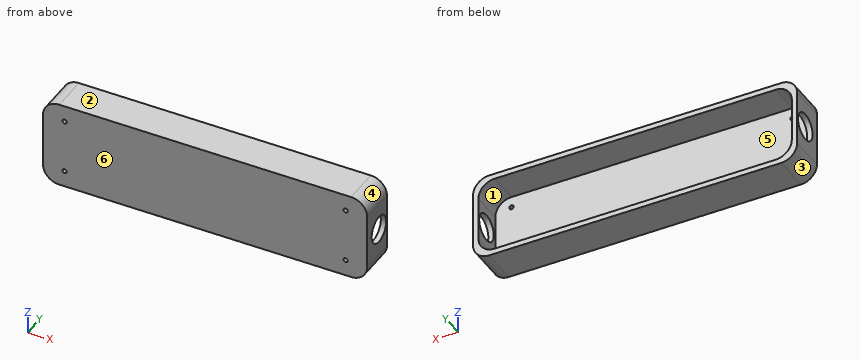
from build123d import *

# Parameters (mm, degrees)
SKETCH1_W               = 300
SKETCH1_H               = 80.5
SKETCH1_W_2             = 290
SKETCH1_H_2             = 70.5
BOSS_EXTRUDE1_DEPTH     = 34
SKETCH1_3_W             = 290
SKETCH1_3_H             = 70.5
BOSS_EXTRUDE2_DEPTH     = 5
FILLET1_R               = 15
FILLET2_R               = 15
FILLET3_R               = 15
FILLET4_R               = 15
FILLET5_R               = 15
FILLET6_R               = 15
FILLET7_R               = 15
FILLET8_R               = 15
SKETCH2_R               = 2
CUT_EXTRUDE1_DEPTH      = 159.984472512
MIRROR2_COPY_1_SKETCH_R = 2
MIRROR2_COPY_1_DEPTH    = 159.984472512
SKETCH3_R               = 12.5
CUT_EXTRUDE2_DEPTH      = 305.591632354


with BuildPart() as part:
    # Sketch1 → Boss-Extrude1 (new body)
    with BuildSketch(Plane(origin=(0, 0, 0), x_dir=(1, 0, 0), z_dir=(0, 1, 0))):
        Rectangle(SKETCH1_W, SKETCH1_H)
        Rectangle(SKETCH1_W_2, SKETCH1_H_2, mode=Mode.SUBTRACT)
    extrude(amount=BOSS_EXTRUDE1_DEPTH)

    # Sketch1_3 → Boss-Extrude2 (add)
    with BuildSketch(Plane(origin=(0, 0, 0), x_dir=(1, 0, 0), z_dir=(0, 1, 0))):
        Rectangle(SKETCH1_3_W, SKETCH1_3_H)
    extrude(amount=BOSS_EXTRUDE2_DEPTH)

    # Fillet1
    fillet1_edges = [part.edges().sort_by_distance(p)[0] for p in [
        (-150, 17, 40.25),
    ]]
    fillet(fillet1_edges, radius=FILLET1_R)

    # Fillet2
    fillet2_edges = [part.edges().sort_by_distance(p)[0] for p in [
        (-150, 17, -40.25),
    ]]
    fillet(fillet2_edges, radius=FILLET2_R)

    # Fillet3
    fillet3_edges = [part.edges().sort_by_distance(p)[0] for p in [
        (150, 17, -40.25),
    ]]
    fillet(fillet3_edges, radius=FILLET3_R)

    # Fillet4
    fillet4_edges = [part.edges().sort_by_distance(p)[0] for p in [
        (150, 17, 40.25),
    ]]
    fillet(fillet4_edges, radius=FILLET4_R)

    # Fillet5
    fillet5_edges = [part.edges().sort_by_distance(p)[0] for p in [
        (-145, 19.5, -35.25),
    ]]
    fillet(fillet5_edges, radius=FILLET5_R)

    # Fillet6
    fillet6_edges = [part.edges().sort_by_distance(p)[0] for p in [
        (-145, 19.5, 35.25),
    ]]
    fillet(fillet6_edges, radius=FILLET6_R)

    # Fillet7
    fillet7_edges = [part.edges().sort_by_distance(p)[0] for p in [
        (145, 19.5, -35.25),
    ]]
    fillet(fillet7_edges, radius=FILLET7_R)

    # Fillet8
    fillet8_edges = [part.edges().sort_by_distance(p)[0] for p in [
        (145, 19.5, 35.25),
    ]]
    fillet(fillet8_edges, radius=FILLET8_R)

    # Sketch2 → Cut-Extrude1 (cut, through all)
    with BuildSketch(Plane(origin=(0, 0, 0), x_dir=(-1, 0, 0), z_dir=(0, -1, 0))):
        with Locations(Location((-130, -25, 0), (0, 0, 90))):
            Circle(SKETCH2_R)
    cut_extrude1 = extrude(amount=-CUT_EXTRUDE1_DEPTH, mode=Mode.SUBTRACT)

    # Mirror1: Cut-Extrude1 across plane
    add(cut_extrude1.mirror(Plane.XY), mode=Mode.SUBTRACT)

    # Mirror2: Cut-Extrude1 across plane
    add(cut_extrude1.mirror(Plane(origin=(0, 0, 0), x_dir=(0, 0, 1), z_dir=(1, 0, 0))), mode=Mode.SUBTRACT)

    # Mirror2 copy 1 sketch → Mirror2 copy 1 (cut, through all)
    with BuildSketch(Plane.XZ):
        with Locations(Location((-130, -25, 0), (0, 0, 90))):
            Circle(MIRROR2_COPY_1_SKETCH_R)
    extrude(amount=-MIRROR2_COPY_1_DEPTH, mode=Mode.SUBTRACT)

    # Sketch3 → Cut-Extrude2 (cut, through all)
    with BuildSketch(Plane(origin=(150, 0, 0), x_dir=(0, 0, -1), z_dir=(1, 0, 0))):
        with Locations((0, 20.125)):
            Circle(SKETCH3_R)
    extrude(amount=-CUT_EXTRUDE2_DEPTH, mode=Mode.SUBTRACT)


solid = part.part
Verification items for the finished model (mm, model axes). Face numbers are marked on the shaded views. A direction names the side the tool comes from. Round coordinates to 2 decimals unless told otherwise and drop trailing zeros. Loops run counter-clockwise (first coordinate to the right, second up) from the corner with the lowest first, then second, coordinate; pieces in that order, holes last. Notation, with made-up numbers: (84.25, 85.5) - (102.25, 85.5) arc R26 cw to (102.25, 116.5) - close; hole circle Ø3 at (14, -35.75). An arc over 180 degrees is marked (long way). Answer in a Markdown table with one row per item. Add a question column.
Q1. Tool access check on the marked faces 5 and 6. Record the directions out of +Z, -Z, +X, -X, +Y, -Y that give a thin tool (end or side, any length) a straight path to the whole face; none if there is none.
Q2. Gauge pin test, flat ends, axial feed: pin 1 (1.5 mm diameter, centred on y = 4, z = -31.5, fed in from +X); pin 2 (21 mm diameter, centred on x = -13.5, z = -11, fed in from +Y); pin 3 (3.5 mm diameter, centred on x = -130, z = 25, fed in from +Y). Record the tip position at first contact, or that the pin passes through.
Q3. Section check C-C on y = 12. Enter the section's corners in (x, z), plus the area to 3 significant figures.
Q4. Section check D-D on z = 32. Enter the section's corners in (x, y).
Q5. Section check A-A on z = 0. Enter the section's corners in (x, y) (3 decimals), plus the area to 3 significant figures.
Q6. Release check for a two-part mould opening along X. For the marked faces 1, 2, 3 and 4 record: pulls with the +X half, pulls with the -X half, needs draft (parallel to the pull), parting line crosses it, or undercut.
Q7. Section check B-B on x = -3.5. Enter the section's corners in (y, z), plus the area to 4 significant figures.
Q8. Material ranges on line 1 (Z direction, x = 130, y = 2.15); line 2 (X direction, y = 3, z = -25); line 3 (Z direction, x = -54, y = 17), recorded low to high.
Found:
| question | item | result |
|---|---|---|
| 1 | face 5 | +Y |
| 1 | face 6 | +Z, -Z, +X, -X, -Y |
| 2 | pin 1 | stops at x = 148.96 |
| 2 | pin 2 | stops at y = 5 |
| 2 | pin 3 | passes through |
| 3 | outline | (-150, -25.25) arc R15 ccw to (-135, -40.25) - (135, -40.25) arc R15 ccw to (150, -25.25) - (150, -9.5) - (145, -9.5) - (145, -20.25) arc R15 cw to (130, -35.25) - (-130, -35.25) arc R15 cw to (-145, -20.25) - (-145, -9.5) - (-150, -9.5) - close; (-150, 9.5) - (-145, 9.5) - (-145, 20.25) arc R15 cw to (-130, 35.25) - (130, 35.25) arc R15 cw to (145, 20.25) - (145, 9.5) - (150, 9.5) - (150, 25.25) arc R15 ccw to (135, 40.25) - (-135, 40.25) arc R15 ccw to (-150, 25.25) - close |
| 3 | area | 3,520 mm² |
| 4 | outline | (-148.4, 0) - (148.4, 0) - (148.4, 34) - (139.32, 34) - (139.32, 5) - (-139.32, 5) - (-139.32, 34) - (-148.4, 34) - close |
| 5 | outline | (-150, 0) - (150, 0) - (150, 7.625) - (145, 7.625) - (145, 5) - (-145, 5) - (-145, 7.625) - (-150, 7.625) - close; (-150, 32.625) - (-145, 32.625) - (-145, 34) - (-150, 34) - close; (145, 32.625) - (150, 32.625) - (150, 34) - (145, 34) - close |
| 5 | area | 1,540 mm² |
| 6 | face 1 | undercut |
| 6 | face 2 | needs draft |
| 6 | face 3 | pulls with the -X half |
| 6 | face 4 | pulls with the +X half |
| 7 | outline | (0, -40.25) - (34, -40.25) - (34, -35.25) - (5, -35.25) - (5, 35.25) - (34, 35.25) - (34, 40.25) - (0, 40.25) - close |
| 7 | area | 692.5 mm² |
| 8 | line 1 | z = -40.25 to -27, -23 to 23, 27 to 40.25 |
| 8 | line 2 | x = -150 to -132, -128 to 128, 132 to 150 |
| 8 | line 3 | z = -40.25 to -35.25, 35.25 to 40.25 |
